For this review, take the finished solid that the model builds, in its own axes (mm). Face numbers are marked on the shaded views. A direction names the side the tool comes from. Give positions to 0.01 mm unless a question says otherwise; leave off trailing zeros. Write each loop counter-clockwise with the first axis right and the second up, starting at its lowest first coordinate (ties: lowest second). Pieces come first, ordered by that corner, then holes. Notation, with made-up numbers: (17.25, 67.5) -> (59.25, 67.5) arc R17 ccw to (59.25, 89.5) -> close; hole circle Ø5 at (-27.5, 42). An arc over 180 degrees is marked (long way). Return JSON: item names as keys, results as strings.
from build123d import *

# Parameters (mm, degrees)
F0_R     = 12.7
F1_DEPTH = 25.4
F2_R     = 12.7
F3_DEPTH = 25.4
F4_R     = 12.7


with BuildPart() as f1:
    # F0 (on Front) → F1 (new body)
    with BuildSketch(Plane.XZ):
        with BuildLine():
            Line((61.220638, -15.7988), (-25.29539, 43.611169))
            ThreePointArc((-25.29539, 43.611169), (-51.969765, 45.176223), (-65.779362, 22.3012))
            Line((-65.779362, 22.3012), (-65.779362, -28.4988))
            Line((-65.779362, -28.4988), (61.220638, -28.4988))
            Line((61.220638, -28.4988), (61.220638, -15.7988))
        make_face()
        with Locations((-39.928801, 22.3012)):
            Circle(F0_R, mode=Mode.SUBTRACT)
    extrude(amount=F1_DEPTH)

    # F2 (on face) → F3 (join)
    with BuildSketch(Plane.XZ.offset(25.4)):
        with BuildLine():
            Line((61.220638, -28.4988), (61.220638, -15.7988))
            Line((61.220638, -15.7988), (-14.078241, -15.7988))
            Line((-14.078241, -15.7988), (-14.078241, 22.3012))
            ThreePointArc((-14.078241, 22.3012), (-17.053778, 34.342163), (-25.29539, 43.611169))
            ThreePointArc((-25.29539, 43.611169), (-51.969765, 45.176223), (-65.779362, 22.3012))
            Line((-65.779362, 22.3012), (-65.779362, -15.7988))
            Line((-65.779362, -15.7988), (-65.779362, -28.4988))
            Line((-65.779362, -28.4988), (61.220638, -28.4988))
        make_face()
        with Locations((-39.928801, 22.3012)):
            Circle(F2_R, mode=Mode.SUBTRACT)
    extrude(amount=F3_DEPTH)

    # F4
    f4_edges = [f1.edges().sort_by_distance(p)[0] for p in [
        (61.220638, -50.8, -22.1488),
    ]]
    fillet(f4_edges, radius=F4_R)


solid = f1.part
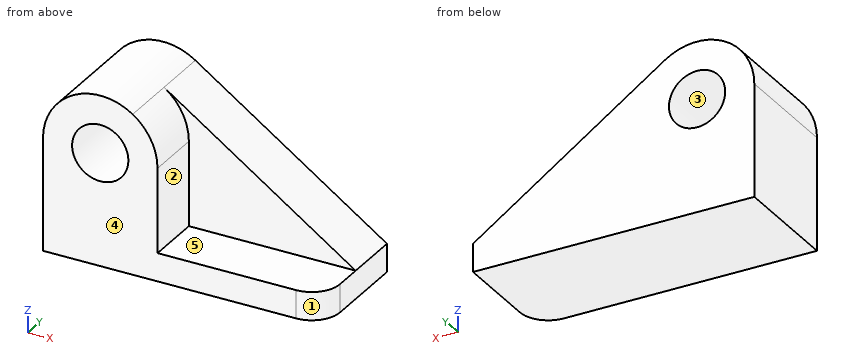
1. For pin 1 (20.5 mm diameter, centred on y = -40, z = -3, fed in from +X); pin 2 (1 mm diameter, centred on y = -7.5, z = -3.5, fed in from +X); pin 3 (18 mm diameter, centred on x = 6.5, z = 7, fed in from -Y), all flat-tipped, find the tip position at first contact; note any pin that passes through.
Results found:
{"pin 1": "stops at x = -14.08", "pin 2": "stops at x = 44.04", "pin 3": "stops at y = -25.4"}
2. Add section C-C, the plane z = 16. State the section outline as (x, y) points, plus the area to 3 significant figures.
Results found:
{"outline": "(-65.78, -50.8) -> (-50.96, -50.8) -> (-50.96, 0) -> (-65.78, 0) -> close; (-28.9, -50.8) -> (-14.08, -50.8) -> (-14.08, -25.4) -> (14.91, -25.4) -> (14.91, 0) -> (-28.9, 0) -> close", "area": "2,240 mm²"}
3. Add section D-D, the plane y = -19.5. State the section outline as (x, z) points, plus the area to 3 significant figures.
Results found:
{"outline": "(-65.78, -28.5) -> (61.22, -28.5) -> (61.22, -15.8) -> (-25.3, 43.61) arc R25.85 ccw to (-65.78, 22.3) -> close; hole circle Ø25.4 at (-39.93, 22.3)", "area": "6,100 mm²"}
4. To check wall thickness, follow probe 1 along Y at (x, z) = (-10.5, 8.5); probe 2 along X at (y, z) = (-40.5, -2); probe 3 along Z at (x, y) = (21.5, -43.5). State the ranges of each line that lie inside material, in increasing order.
Results found:
{"probe 1": "y = -25.4 to 0", "probe 2": "x = -65.78 to -14.08", "probe 3": "z = -28.5 to -15.8"}
5. The part is to be moulded in two halves that separate along Z. For the marked faces 3, 4 and 5, say which applies: +Z half, -Z half, draft (parallel to the pull), parting line (faces both ways), or undercut.
Results found:
{"face 3": "undercut", "face 4": "draft", "face 5": "+Z half"}
6. Add section A-A, the plane y = -33.5. State the section outline as (x, z) points, plus the area to 3 significant figures.
Results found:
{"outline": "(-65.78, -28.5) -> (61.22, -28.5) -> (61.22, -15.8) -> (-14.08, -15.8) -> (-14.08, 22.3) arc R25.85 ccw to (-25.3, 43.61) arc R25.85 ccw to (-65.78, 22.3) -> close; hole circle Ø25.4 at (-39.93, 22.3)", "area": "4,130 mm²"}
7. For the marked faces 1 and 2, list the 3-axis set-ups (+Z, -Z, +X, -X, +Y, -Y) from which the entire face can be reached by the end or side of a thin tool; tool diameter is ignored.
Results found:
{"face 1": "+Z, -Z, +X, -Y", "face 2": "+Z, +X, -Y"}
8. Add section B-B, the plane x = -51. State the section outline as (y, z) points.
Results found:
{"outline": "(-50.8, -28.5) -> (0, -28.5) -> (0, 16.08) -> (-50.8, 16.08) -> close; (-50.8, 28.52) -> (0, 28.52) -> (0, 45.66) -> (-50.8, 45.66) -> close"}
